Geometry: final body of the model. Coordinates: model frame, mm. A direction names the side the tool comes from. Give positions to 0.01 mm unless a question says otherwise; leave off trailing zeros. Order: outer loops, then holes, each group sorted by start corner. A loop starts at its lowest first (then second) coordinate and runs counter-clockwise, first axis right, second up. Notation, with made-up numbers: (38, 48) -> (84, 48) arc R20 ccw to (84, 63) -> close; hole circle Ø8 at (41.5, 6). An arc over 180 degrees is marked (long way). Answer in a Markdown table with one row per item. Add a question column.
Q1. Cut plane C-C on x = 79. Return the cut outline in (y, z), and give its area (3 significant figures).
Q2. Set-up query: faces 1 (the face through (-4.617, -3, -16)), 2 (the face through (-15.86, -20.52, -36.71)), 3 (the face through (-27, -23.973, -10)). Return all of +Z, -Z, +X, -X, +Y, -Y with unobstructed straight access to the full face (end or side cutting, diameter ignored); none if empty.
Q3. Cut plane A-A on z = -18. Return the cut outline in (x, y), and give its area (3 significant figures).
Q4. Pull-direction query (Y, two-part tool) for faces 4 (the face through (45, -3, 0)), 5 (the face through (-15.9, -2.1, -36.7)), 6 (the face through (-27, 21.747, 1)); classes: +Y half, -Y half, draft (parallel to the pull), parting line (faces both ways), or undercut.
Q5. Cut plane B-B on y = 13.5. Return the cut outline in (x, z).
Q6. Line query: line 1 along X through (y, z) = (15.5, -19); line 2 along Y through (x, z) = (-10, -26.5); line 3 along X through (y, z) = (16, -22). Output: solid intervals per line, ascending. Write a range as from..to.
Q7. Contact query for flat-ended pins moving along their axis: P1, Ø2, axis at y = 4.5, z = -35.5, coming from the +X side; P2, Ø23, axis at x = -27.46, z = -18.14, coming from the +Y side; P3, Ø3, axis at y = -9, z = -42, coming from the +X side. Output: stop coordinate, or through.
Q8. Cut plane D-D on z = -8. Return the cut outline in (x, y).
from build123d import *

# Parameters (mm, degrees)
SKETCH1_W                           = 247.65
SKETCH1_H                           = 50.8
BOSS_EXTRUDE1_DEPTH                 = 10.16
CUT_EXTRUDE1_DEPTH                  = 160.914701011
CUT_EXTRUDE1_DEPTH_BACK             = 160.914701011
SKETCH7_R                           = 22.847252038
BOSS_EXTRUDE2_DEPTH                 = 50.8
SKETCH8_R                           = 18.9865
CUT_EXTRUDE2_DEPTH                  = 45.72
SKETCH9_R                           = 7.9375
CUT_EXTRUDE3_DEPTH                  = 164.275821461
BOSS_EXTRUDE3_DEPTH                 = 50.8
BOSS_EXTRUDE4_START                 = -50.8
BOSS_EXTRUDE4_DEPTH                 = 50.8
BOSS_EXTRUDE5_START                 = -50.8
BOSS_EXTRUDE5_DEPTH                 = 50.8
SKETCH22_W                          = 30.1625
SKETCH22_H                          = 50.8
BOSS_EXTRUDE6_DEPTH                 = 2.54
CUT_EXTRUDE4_DEPTH                  = 166.420598915
TAP_DRILL_FOR_1_4_HELICOIL1_REACH   = 172.648
TAP_DRILL_FOR_1_4_HELICOIL1_BORE_R  = 3.3782
CUT_EXTRUDE5_DEPTH                  = 5.55625
CUT_EXTRUDE5_DIRECTION_2_REACH      = 168.46
CUT_EXTRUDE5_DIRECTION_2_END_RADIUS = 18.9865


with BuildPart() as part:
    # Sketch1 → Boss-Extrude1 (new body)
    with BuildSketch(Plane.XY):
        with Locations((-27.465601161, -3.653036721)):
            Rectangle(SKETCH1_W, SKETCH1_H)
    extrude(amount=BOSS_EXTRUDE1_DEPTH)

    # Sketch6 → Cut-Extrude1 (cut, two sides: drawn at the far end of the back side and taken through both)
    with BuildSketch(Plane(origin=(0, 21.746963279, 0), x_dir=(1, 0, 0), z_dir=(0, 1, 0)).offset(-CUT_EXTRUDE1_DEPTH_BACK)):
        with BuildLine():
            Line((211.371578383, 140.927334364), (-20.861601161, 0))
            ThreePointArc((-20.861601161, 0), (-27.465601161, -1.847030056), (-34.069601161, 0))
            Line((-34.069601161, 0), (-266.302780705, 140.927334364))
            Line((-266.302780705, 140.927334364), (-266.302780705, 684.223803161))
            Line((-266.302780705, 684.223803161), (211.371578383, 684.223803161))
            Line((211.371578383, 684.223803161), (211.371578383, 140.927334364))
        make_face()
    extrude(amount=CUT_EXTRUDE1_DEPTH + CUT_EXTRUDE1_DEPTH_BACK, mode=Mode.SUBTRACT)

    # Sketch7 → Boss-Extrude2 (add, through all)
    with BuildSketch(Plane(origin=(0, 21.746963279, 0), x_dir=(1, 0, 0), z_dir=(0, 1, 0))):
        with Locations((-27.464264218, 18.13847077)):
            Circle(SKETCH7_R)
    extrude(amount=-BOSS_EXTRUDE2_DEPTH)

    # Sketch8 → Cut-Extrude2 (cut)
    with BuildSketch(Plane(origin=(0, 21.746963279, 0), x_dir=(1, 0, 0), z_dir=(0, 1, 0))):
        with Locations(Location((-27.464264218, 18.13847077, 0), (0, 0, 270))):
            Circle(SKETCH8_R)
    extrude(amount=-CUT_EXTRUDE2_DEPTH, mode=Mode.SUBTRACT)

    # Sketch9 → Cut-Extrude3 (cut, through all)
    with BuildSketch(Plane(origin=(0, -23.973036721, 0), x_dir=(1, 0, 0), z_dir=(0, 1, 0))):
        with Locations(Location((-27.464264218, 18.13847077, 0), (0, 0, 270))):
            Circle(SKETCH9_R)
    extrude(amount=-CUT_EXTRUDE3_DEPTH, mode=Mode.SUBTRACT)

    # Sketch12 → Boss-Extrude3 (add)
    with BuildSketch(Plane(origin=(0, 21.746963279, 0), x_dir=(1, 0, 0), z_dir=(0, 1, 0))):
        with BuildLine():
            Line((-4.61701218, 18.13847077), (-4.61701218, 0))
            Line((-4.61701218, 0), (-13.572079227, 0))
            ThreePointArc((-13.572079227, 0), (-6.977742093, 8.024157302), (-4.61701218, 18.13847077))
        make_face()
        with BuildLine():
            Line((-50.311516256, 18.13847077), (-50.311516256, 0))
            Line((-50.311516256, 0), (-41.356449209, 0))
            ThreePointArc((-41.356449209, 0), (-47.950786342, 8.024157302), (-50.311516256, 18.13847077))
        make_face()
    extrude(amount=-BOSS_EXTRUDE3_DEPTH)

    # Sketch16 → Boss-Extrude4 (add)
    with BuildSketch(Plane.XZ.offset(29.053036721).offset(BOSS_EXTRUDE4_START)):
        with BuildLine():
            Line((-50.311516256, -18.13847077), (-50.311516256, -40.985722808))
            Line((-50.311516256, -40.985722808), (-27.464264218, -40.985722808))
            ThreePointArc((-27.464264218, -40.985722808), (-43.619711065, -34.293917617), (-50.311516256, -18.13847077))
        make_face()
    extrude(amount=BOSS_EXTRUDE4_DEPTH)

    # Sketch18 → Boss-Extrude5 (add)
    with BuildSketch(Plane.XZ.offset(29.053036721).offset(BOSS_EXTRUDE5_START)):
        with BuildLine():
            Line((-4.61701218, -18.13847077), (-4.61701218, -40.985722808))
            Line((-4.61701218, -40.985722808), (-27.464264218, -40.985722808))
            ThreePointArc((-27.464264218, -40.985722808), (-11.30881737, -34.293917617), (-4.61701218, -18.13847077))
        make_face()
    extrude(amount=BOSS_EXTRUDE5_DEPTH)

    # Sketch22 → Boss-Extrude6 (add)
    with BuildSketch(Plane(origin=(0, 0, -40.985722808), x_dir=(-1, 0, 0), z_dir=(0, 0, -1))):
        with Locations((27.451516256, -3.653036721)):
            Rectangle(SKETCH22_W, SKETCH22_H)
    extrude(amount=BOSS_EXTRUDE6_DEPTH)

    # Sketch23 → Cut-Extrude4 (cut, through all)
    with BuildSketch(Plane(origin=(0, 21.746963279, 0), x_dir=(1, 0, 0), z_dir=(0, 1, 0))):
        Polygon((-42.532766256, 40.985722808), (-50.311516256, 33.206972808), (-50.311516256, 40.985722808), align=None)
        Polygon((-12.370266256, 40.985722808), (-4.61701218, 33.232468732), (-4.61701218, 40.985722808), align=None)
    extrude(amount=-CUT_EXTRUDE4_DEPTH, mode=Mode.SUBTRACT)

    # Tap Drill for 1/4 Helicoil1 bore → Tap Drill for 1/4 Helicoil1 (cut, up to next)
    with BuildSketch(Plane(origin=(14.307728276, 0, -14.307728276), x_dir=(-0.7071067811865561, 0, -0.7071067811865389), z_dir=(0.7071067811865389, 0, -0.7071067811865561)), mode=Mode.PRIVATE) as tap_drill_for_1_4_helicoil1_sk1:
        with Locations((32.224624617, -4.923054714)):
            Circle(TAP_DRILL_FOR_1_4_HELICOIL1_BORE_R)
    tap_drill_for_1_4_helicoil1_tool1 = extrude(tap_drill_for_1_4_helicoil1_sk1.sketch, amount=-TAP_DRILL_FOR_1_4_HELICOIL1_REACH, mode=Mode.PRIVATE) & part.part
    # Tap Drill for 1/4 Helicoil1 bore → Tap Drill for 1/4 Helicoil1 (cut, up to next)
    with BuildSketch(Plane(origin=(14.307728276, 0, -14.307728276), x_dir=(-0.7071067811865561, 0, -0.7071067811865389), z_dir=(0.7071067811865389, 0, -0.7071067811865561)), mode=Mode.PRIVATE) as tap_drill_for_1_4_helicoil1_sk2:
        with Locations((32.24600315, -17.623036721)):
            Circle(TAP_DRILL_FOR_1_4_HELICOIL1_BORE_R)
    tap_drill_for_1_4_helicoil1_tool2 = extrude(tap_drill_for_1_4_helicoil1_sk2.sketch, amount=-TAP_DRILL_FOR_1_4_HELICOIL1_REACH, mode=Mode.PRIVATE) & part.part
    add(tap_drill_for_1_4_helicoil1_tool1.solids().sort_by_distance((-8.478522, -4.923055, -37.093979))[0], mode=Mode.SUBTRACT)
    add(tap_drill_for_1_4_helicoil1_tool2.solids().sort_by_distance((-8.493639, -17.623037, -37.109096))[0], mode=Mode.SUBTRACT)

    # Sketch28 → Cut-Extrude5 (cut)
    with BuildSketch(Plane(origin=(8.919574603, 0, -8.919574603), x_dir=(-0.7071067811865561, 0, -0.7071067811865389), z_dir=(0.7071067811865389, 0, -0.7071067811865561))):
        Polygon((28.946446362, -23.338036721), (35.545559939, -23.338036721), (38.845116727, -17.623036721), (35.545559939, -11.908036721), (28.946446362, -11.908036721), (25.646889574, -17.623036721), align=None)
        Polygon((38.823738194, -4.923054714), (35.524181405, 0.791945286), (28.925067829, 0.791945286), (25.62551104, -4.923054714), (28.925067829, -10.638054714), (35.524181405, -10.638054714), align=None)
    extrude(amount=CUT_EXTRUDE5_DEPTH, mode=Mode.SUBTRACT)

    # Cut-Extrude5 direction 2: up to this cylinder (the profile starts outside it)
    cut_extrude5_direction_2_end = Plane(origin=(-27.464264218, -11.273046, -18.13847077), z_dir=(0, 1, 0)) * Cylinder(CUT_EXTRUDE5_DIRECTION_2_END_RADIUS, 388.592982, mode=Mode.PRIVATE)
    # Sketch28 → Cut-Extrude5 direction 2 (cut, up to the surface)
    with BuildSketch(Plane(origin=(8.919574603, 0, -8.919574603), x_dir=(-0.7071067811865561, 0, -0.7071067811865389), z_dir=(0.7071067811865389, 0, -0.7071067811865561)), mode=Mode.PRIVATE) as cut_extrude5_direction_2_sk1:
        Polygon((28.946446362, -23.338036721), (35.545559939, -23.338036721), (38.845116727, -17.623036721), (35.545559939, -11.908036721), (28.946446362, -11.908036721), (25.646889574, -17.623036721), align=None)
    cut_extrude5_direction_2_tool1 = extrude(cut_extrude5_direction_2_sk1.sketch, amount=-CUT_EXTRUDE5_DIRECTION_2_REACH, mode=Mode.PRIVATE) - cut_extrude5_direction_2_end
    add(cut_extrude5_direction_2_tool1.solids().sort_by_distance((-13.881793, -17.623037, -31.720942))[0], mode=Mode.SUBTRACT)
    # Sketch28 → Cut-Extrude5 direction 2 (cut, up to the surface)
    with BuildSketch(Plane(origin=(8.919574603, 0, -8.919574603), x_dir=(-0.7071067811865561, 0, -0.7071067811865389), z_dir=(0.7071067811865389, 0, -0.7071067811865561)), mode=Mode.PRIVATE) as cut_extrude5_direction_2_sk2:
        Polygon((38.823738194, -4.923054714), (35.524181405, 0.791945286), (28.925067829, 0.791945286), (25.62551104, -4.923054714), (28.925067829, -10.638054714), (35.524181405, -10.638054714), align=None)
    cut_extrude5_direction_2_tool2 = extrude(cut_extrude5_direction_2_sk2.sketch, amount=-CUT_EXTRUDE5_DIRECTION_2_REACH, mode=Mode.PRIVATE) - cut_extrude5_direction_2_end
    add(cut_extrude5_direction_2_tool2.solids().sort_by_distance((-13.866676, -4.923055, -31.705825))[0], mode=Mode.SUBTRACT)


solid = part.part
Completed:
| question | item | result |
|---|---|---|
| 1 | outline | (-29.05, 0) -> (21.75, 0) -> (21.75, 10.16) -> (-29.05, 10.16) -> close |
| 1 | area | 516 mm² |
| 2 | face 1 | -Z, +X, +Y, -Y |
| 2 | face 2 | none |
| 2 | face 3 | +Y |
| 3 | outline | (-50.31, -29.05) -> (-35.4, -29.05) -> (-35.4, -23.97) -> (-46.45, -23.97) -> (-46.45, 21.75) -> (-50.31, 21.75) -> close; (-19.53, -29.05) -> (-4.62, -29.05) -> (-4.62, 21.75) -> (-8.48, 21.75) -> (-8.48, -23.97) -> (-19.53, -23.97) -> close |
| 3 | area | 505 mm² |
| 4 | face 4 | draft |
| 4 | face 5 | undercut |
| 4 | face 6 | +Y half |
| 5 | outline | (-151.29, 0) -> (-50.31, 0) -> (-50.31, -33.21) -> (-42.53, -40.99) -> (-42.53, -43.53) -> (-12.37, -43.53) -> (-12.37, -40.99) -> (-4.62, -33.23) -> (-4.62, 0) -> (96.36, 0) -> (96.36, 10.16) -> (-151.29, 10.16) -> close; hole circle Ø37.97 at (-27.46, -18.14) |
| 6 | line 1 | x = -50.31..-46.43, -8.5..-4.62 |
| 6 | line 2 | y = -29.05..-17.9, -17.34..-5.24, -4.6..21.75 |
| 6 | line 3 | x = -50.31..-46.05, -8.87..-4.62 |
| 7 | P1 | stops at x = -5.88 |
| 7 | P2 | stops at y = -23.97 |
| 7 | P3 | stops at x = -11.88 |
| 8 | outline | (-50.31, -29.05) -> (-4.62, -29.05) -> (-4.62, 21.75) -> (-11.41, 21.75) -> (-11.41, -23.97) -> (-43.52, -23.97) -> (-43.52, 21.75) -> (-50.31, 21.75) -> close |
